from build123d import *

# Parameters (mm, degrees)
SKETCH007_W                 = 31.8
SKETCH007_H                 = 31.8
PAD006_DEPTH                = 1
SKETCH009_W                 = 15
SKETCH009_H                 = 25.4
POCKET001_DEPTH             = 1.001
SKETCH010_R                 = 2.032
SKETCH010_R_2               = 1.232
PAD008_DEPTH                = 9.2
SKETCH010_MIRRORED009_2_R   = 2.032
SKETCH010_MIRRORED009_2_R_2 = 1.232
PAD008_MIRRORED009_2_DEPTH  = 9.2
SKETCH027_W                 = 31.8
SKETCH027_H                 = 31.8
SKETCH027_W_2               = 29.4
SKETCH027_H_2               = 29.4
PAD016_DEPTH                = 14
PAD017_DEPTH                = 5.3
PAD017_MIRRORED025_2_DEPTH  = 5.3
SKETCH029_W                 = 9
SKETCH029_H                 = 1.5
SKETCH029_W_2               = 16
POCKET010_DEPTH             = 9.6
SKETCH030_W                 = 1.5
SKETCH030_H                 = 9
POCKET011_DEPTH             = 9.6
FILLET013_R                 = 2
BODY002_PLACEMENT_ANGLE     = 180


with BuildPart() as part:
    # Sketch007 → Pad006 (new body)
    with BuildSketch(Plane.XY):
        Rectangle(SKETCH007_W, SKETCH007_H)
    extrude(amount=PAD006_DEPTH)

    # Sketch009 → Pocket001 (cut, through all)
    with BuildSketch(Plane.XY.offset(1)):
        Rectangle(SKETCH009_W, SKETCH009_H)
    extrude(amount=-POCKET001_DEPTH, mode=Mode.SUBTRACT)

    # Sketch010 (on Face5 of Pocket001) → Pad008 (join)
    with BuildSketch(Plane.XY.offset(1)):
        with Locations((10.16, 10.16)):
            Circle(SKETCH010_R)
        with Locations((10.16, 10.16)):
            Circle(SKETCH010_R_2, mode=Mode.SUBTRACT)
    pad008 = extrude(amount=PAD008_DEPTH)

    # Sketch010 Mirrored009 2 → Pad008 Mirrored009 2 (add)
    with BuildSketch(Plane(origin=(0, 0, 1), x_dir=(-1, 0, 0), z_dir=(0, 0, -1))):
        with Locations((10.16, 10.16)):
            Circle(SKETCH010_MIRRORED009_2_R)
        with Locations((10.16, 10.16)):
            Circle(SKETCH010_MIRRORED009_2_R_2, mode=Mode.SUBTRACT)
    pad008_mirrored009_2 = extrude(amount=-PAD008_MIRRORED009_2_DEPTH)

    # Mirrored010: Pad008, Pad008 Mirrored009 2 across Sketch010 H_Axis
    add(pad008.mirror(Plane(origin=(0, 0, 1), x_dir=(0, 0, 1), z_dir=(0, 1, 0))))
    add(pad008_mirrored009_2.mirror(Plane(origin=(0, 0, 1), x_dir=(0, 0, 1), z_dir=(0, 1, 0))))

    # Sketch027 (on Face5 of MultiTransform006) → Pad016 (join)
    with BuildSketch(Plane.XY.offset(1)):
        Rectangle(SKETCH027_W, SKETCH027_H)
        Rectangle(SKETCH027_W_2, SKETCH027_H_2, mode=Mode.SUBTRACT)
    extrude(amount=PAD016_DEPTH)

    # Sketch028 (on Face14 of Pad016) → Pad017 (join)
    with BuildSketch(Plane.XZ.offset(15.9)):
        with BuildLine():
            Line((-14.7, 13), (-14.7, 15))
            Line((-14.7, 15), (-14.401415, 14.573576))
            ThreePointArc((-14.401415, 13.426424), (-14.220567, 14), (-14.401415, 14.573576))
            Line((-14.401415, 13.426424), (-14.7, 13))
        make_face()
    pad017 = extrude(amount=-PAD017_DEPTH)

    # Sketch028 Mirrored025 2 → Pad017 Mirrored025 2 (add)
    with BuildSketch(Plane(origin=(0, -15.9, 0), x_dir=(-1, 0, 0), z_dir=(0, 1, 0))):
        with BuildLine():
            Line((-14.7, 13), (-14.7, 15))
            Line((-14.7, 15), (-14.401415, 14.573576))
            ThreePointArc((-14.401415, 13.426424), (-14.220567, 14), (-14.401415, 14.573576))
            Line((-14.401415, 13.426424), (-14.7, 13))
        make_face()
    pad017_mirrored025_2 = extrude(amount=PAD017_MIRRORED025_2_DEPTH)

    # Mirrored026: Pad017, Pad017 Mirrored025 2 across XZ
    add(pad017.mirror(Plane.XZ))
    add(pad017_mirrored025_2.mirror(Plane.XZ))

    # Sketch029 (on Face23 of MultiTransform012) → Pocket010 (cut)
    with BuildSketch(Plane.XY.offset(15)):
        with Locations((0, 15.15)):
            Rectangle(SKETCH029_W, SKETCH029_H)
        with Locations((0, -15.15)):
            Rectangle(SKETCH029_W_2, SKETCH029_H)
    extrude(amount=-POCKET010_DEPTH, mode=Mode.SUBTRACT)

    # Sketch030 (on Face18 of Pocket010) → Pocket011 (cut)
    with BuildSketch(Plane.XY.offset(15)):
        with Locations((15.15, 0)):
            Rectangle(SKETCH030_W, SKETCH030_H)
    pocket011 = extrude(amount=-POCKET011_DEPTH, mode=Mode.SUBTRACT)

    # Mirrored027: Pocket011 across Sketch030 V_Axis
    add(pocket011.mirror(Plane(origin=(0, 0, 15), x_dir=(0, 0, 1), z_dir=(1, 0, 0))), mode=Mode.SUBTRACT)

    # Fillet013
    fillet013_edges = [part.edges().sort_by_distance(p)[0] for p in [
        (7.5, 12.7, 0.5),
        (-7.5, 12.7, 0.5),
        (7.5, -12.7, 0.5),
        (-7.5, -12.7, 0.5),
    ]]
    fillet(fillet013_edges, radius=FILLET013_R)


with BuildPart() as part_1:
    # Body002 placement: moved
    add(part.part.moved(Location((0, 0, 15))).rotate(Axis((0, 0, 15), (0, 1, 0)), BODY002_PLACEMENT_ANGLE))


solid = part_1.part
The listing builds one solid part. Answer for the finished solid, in the listing's coordinates (mm). A direction names the side the tool comes from. Coordinates: 2 decimals unless noted, no trailing zeros. Loops run counter-clockwise (first coordinate to the right, second up) from the corner with the lowest first, then second, coordinate; pieces in that order, holes last. Notation, with made-up numbers: (-13, -8) -> (26, -8) arc R17 ccw to (26, 25) -> close; hole circle Ø6 at (18, -26). An arc over 180 degrees is marked (long way). Answer in a Markdown table with one row per item. Add a question column.
1. Flat-ended cylindrical pins translate along their axes: P1, Ø0.7, axis at x = 10, y = -10, coming from the -Z side; P2, Ø4, axis at x = 2, z = 2, coming from the +Y side; P3, Ø1.2, axis at x = 9.5, y = 10, coming from the -Z side; P4, Ø2, axis at x = 6.5, z = 2.5, coming from the -Y side. Find the tip coordinate at first contact, or state that the pin passes through.
2. Determine the mould class of faces 1 (the flat face through (15, -4.5, 5)), 2 (the flat face through (10, 0, 14)), 3 (the flat face through (-15.9, 0, 11)), 4 (the flat face through (14.7, 0, 10)) for opening direction X: +X half, -X half, draft (parallel to the pull), parting line (faces both ways), or undercut.
3. The part is cut by section A-A, the plane z = 12. Count the separate pieces of the cut face and the enclosed holes in it, then the cut area to 3 significant figures.
4. The part is cut by section D-D, the plane x = 10.16. Write down the section's boundary in (y, z).
5. The part is cut by section B-B, the plane y = -5. Write down the section's boundary in (x, z), then the cut area to 3 significant figures.
6. Consider line 1 (Y direction, x = 10.16, z = 10.75); line 2 (X direction, y = -10.5, z = 6.75); line 3 (Y direction, x = -2.5, z = 13). Determine where each line is inside the solid, lowest interval first. Write a range as [from, to].
7. For faces 5 (the flat face through (11, 9, 4.8)), 6 (the flat face through (15, 4.5, 5)), 7 (the flat face through (0, 15, 9.6)), 8 (the flat face through (8, -15, 5)), determine the directions among +Z, -Z, +X, -X, +Y, -Y from which every point of the face is accessible in a straight line to the end or side of a thin tool.
Answer below:
| question | item | result |
|---|---|---|
| 1 | P1 | z = 14 |
| 1 | P2 | through |
| 1 | P3 | z = 4.8 |
| 1 | P4 | y = 14.7 |
| 2 | face 1 | draft |
| 2 | face 2 | undercut |
| 2 | face 3 | -X half |
| 2 | face 4 | undercut |
| 3 | separate pieces | 5 |
| 3 | enclosed holes | 5 |
| 3 | area | 180 mm2 |
| 4 | outline | (-15.9, 0) -> (-14.7, 0) -> (-14.7, 14) -> (-12.19, 14) -> (-12.19, 4.8) -> (-11.39, 4.8) -> (-11.39, 14) -> (-8.93, 14) -> (-8.93, 4.8) -> (-8.13, 4.8) -> (-8.13, 14) -> (8.13, 14) -> (8.13, 4.8) -> (8.93, 4.8) -> (8.93, 14) -> (11.39, 14) -> (11.39, 4.8) -> (12.19, 4.8) -> (12.19, 14) -> (14.7, 14) -> (14.7, 0) -> (15.9, 0) -> (15.9, 15) -> (-15.9, 15) -> close |
| 5 | outline | (-15.9, 0) -> (-14.7, 0) -> (-14.7, 14) -> (-7.5, 14) -> (-7.5, 15) -> (-15.9, 15) -> close; (7.5, 14) -> (14.7, 14) -> (14.7, 0) -> (15.9, 0) -> (15.9, 15) -> (7.5, 15) -> close |
| 5 | area | 50.4 mm2 |
| 6 | line 1 | [-15.9, -14.7], [-12.19, -11.39], [-8.93, -8.13], [8.13, 8.93], [11.39, 12.19], [14.7, 15.9] |
| 6 | line 2 | [-15.9, -14.7], [-12.16, -11.34], [-8.98, -8.16], [8.16, 8.98], [11.34, 12.16], [14.7, 15.9] |
| 6 | line 3 | [-15.9, -14.7], [14.7, 15.9] |
| 7 | face 5 | -Z |
| 7 | face 6 | -Z, +X, -X |
| 7 | face 7 | -Z, +Y, -Y |
| 7 | face 8 | -Z, -Y |
